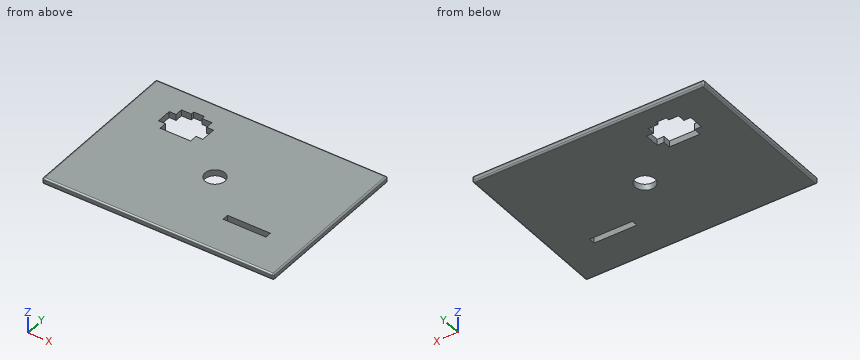
```python
from build123d import *

# Parameters (mm, degrees)
SKETCH1_W           = 75.8
SKETCH1_H           = 53.6
BOSS_EXTRUDE1_DEPTH = 2
SKETCH5_W           = 14
SKETCH5_H           = 2.1
SKETCH5_R           = 3.25
CUT_EXTRUDE1_DEPTH  = 47.461274197
FILLET1_R           = 0.5


with BuildPart() as part:
    # Sketch1 → Boss-Extrude1 (new body)
    with BuildSketch(Plane.XY):
        Rectangle(SKETCH1_W, SKETCH1_H)
    extrude(amount=BOSS_EXTRUDE1_DEPTH)

    # Sketch5 → Cut-Extrude1 (cut, through all)
    with BuildSketch(Plane.XY.offset(2)):
        Polygon((-24.575, 9.475), (-14.575, 9.475), (-14.575, 11.975), (-12.325, 11.975), (-12.325, 16.975), (-14.575, 16.975), (-14.575, 19.475), (-17.825, 19.475), (-17.825, 20.575), (-21.325, 20.575), (-21.325, 19.475), (-24.575, 19.475), (-24.575, 16.975), (-26.825, 16.975), (-26.825, 11.975), (-24.575, 11.975), align=None)
        with Locations((19.575, -13.175)):
            Rectangle(SKETCH5_W, SKETCH5_H)
        Circle(SKETCH5_R)
    extrude(amount=-CUT_EXTRUDE1_DEPTH, mode=Mode.SUBTRACT)

    # Fillet1
    fillet1_edges = [part.edges().sort_by_distance(p)[0] for p in [
        (-37.9, 0, 2),
        (0, -26.8, 2),
        (37.9, 0, 2),
        (0, -26.8, 0),
        (-37.9, 0, 0),
        (0, 26.8, 0),
        (37.9, 0, 0),
        (37.9, -26.8, 1),
        (-37.9, -26.8, 1),
        (-37.9, 26.8, 1),
        (37.9, 26.8, 1),
        (0, 26.8, 2),
    ]]
    fillet(fillet1_edges, radius=FILLET1_R)


solid = part.part
```
Work out the finished part from the listing and answer in its coordinate system (mm). Give positions to 0.01 mm unless a question says otherwise; leave off trailing zeros. Loops run counter-clockwise (first coordinate to the right, second up) from the corner with the lowest first, then second, coordinate; pieces in that order, holes last. Notation, with made-up numbers: (-4.75, 19) -> (41.25, 19) arc R7 cw to (41.25, 29) -> close; hole circle Ø3 at (38, -14.5). An arc over 180 degrees is marked (long way). One line per question, with ' | ' between items. Start each with the question number.
1) This flat-tipped pin is pushed along its axis until it touches: pin 1 (5 mm diameter, centred on x = 0, y = 0, fed in from +Z). Where does it stop, or does it pass through?
2) Section B-B, the plane y = 0 is taken. Determine the outline of the cut face in (x, z).
3) Straight lines are drawn through the part: L1, parallel to Y at x = 0, z = 0.6; L2, parallel to Y at x = -12.5, z = 0.95 (3 decimals); L3, parallel to X at y = 18, z = 1.05 (3 decimals). For each, find the intervals that lie inside material, in ascending order.
4) Section A-A, the plane x = 19 is taken. Determine the outline of the cut face in (y, z) (3 decimals), then the cut area to 3 significant figures.
Resolved:
1) pin 1: through
2) outline: (-37.9, 0.5) arc R0.5 ccw to (-37.4, 0) -> (-3.25, 0) -> (-3.25, 2) -> (-37.4, 2) arc R0.5 ccw to (-37.9, 1.5) -> close; (3.25, 0) -> (37.4, 0) arc R0.5 ccw to (37.9, 0.5) -> (37.9, 1.5) arc R0.5 ccw to (37.4, 2) -> (3.25, 2) -> close
3) L1: -26.8 to -3.25, 3.25 to 26.8 | L2: -26.8 to 11.975, 16.975 to 26.8 | L3: -37.9 to -24.575, -14.575 to 37.9
4) outline: (-26.8, 0.5) arc R0.5 ccw to (-26.3, 0) -> (-14.225, 0) -> (-14.225, 2) -> (-26.3, 2) arc R0.5 ccw to (-26.8, 1.5) -> close; (-12.125, 0) -> (26.3, 0) arc R0.5 ccw to (26.8, 0.5) -> (26.8, 1.5) arc R0.5 ccw to (26.3, 2) -> (-12.125, 2) -> close | area: 103 mm2
